from build123d import *

# Parameters (mm, degrees)
SKETCH1_W                   = 54
SKETCH1_H                   = 65
BOSS_EXTRUDE1_DEPTH         = 65
SKETCH2_W                   = 21
SKETCH2_H                   = 41.5
CUT_EXTRUDE1_DEPTH          = 107.611444039
FILLET1_R                   = 6
SKETCH3_W                   = 21
SKETCH3_H                   = 56
CUT_EXTRUDE2_DEPTH          = 32
CUT_EXTRUDE_THIN3_DEPTH     = 9
CUT_EXTRUDE3_DEPTH          = 9
M3_TAPPED_HOLE1_D           = 2.5
M3_TAPPED_HOLE1_CSINK_D     = 3.05
M3_TAPPED_HOLE1_CSINK_ANGLE = 90
HOLE1_D                     = 6.5
HOLE1_CBORE_D               = 11
HOLE1_CBORE_DEPTH           = 7
EXTRUDE_THIN1_START         = 1.5
EXTRUDE_THIN1_DEPTH         = 1.5
M3_TAPPED_HOLE2_D           = 2.5
M3_TAPPED_HOLE2_CSINK_D     = 3.05
M3_TAPPED_HOLE2_CSINK_ANGLE = 90


with BuildPart() as part:
    # Sketch1 → Boss-Extrude1 (new body)
    with BuildSketch(Plane.XY):
        with Locations((27, 32.5)):
            Rectangle(SKETCH1_W, SKETCH1_H)
    extrude(amount=BOSS_EXTRUDE1_DEPTH)

    # Sketch2 → Cut-Extrude1 (cut, through all)
    with BuildSketch(Plane.XY.offset(65)):
        with Locations((27, 32.5)):
            Rectangle(SKETCH2_W, SKETCH2_H)
    extrude(amount=-CUT_EXTRUDE1_DEPTH, mode=Mode.SUBTRACT)

    # Fillet1
    fillet1_edges = [part.edges().sort_by_distance(p)[0] for p in [
        (0, 65, 32.5),
        (0, 0, 32.5),
        (54, 0, 32.5),
        (54, 65, 32.5),
    ]]
    fillet(fillet1_edges, radius=FILLET1_R)

    # Sketch3 → Cut-Extrude2 (cut)
    with BuildSketch(Plane.XY.offset(65)):
        with Locations((27, 32.5)):
            Rectangle(SKETCH3_W, SKETCH3_H)
    extrude(amount=-CUT_EXTRUDE2_DEPTH, mode=Mode.SUBTRACT)

    # Sketch4 → Cut-Extrude-Thin3 (cut)
    with BuildSketch(Plane.XY.offset(65)):
        with BuildLine():
            Line((6.119863014, 48.642808121), (20.863013699, 55.83321895))
            ThreePointArc((20.863013699, 55.83321895), (27, 57.25), (33.136986301, 55.83321895))
            Line((33.136986301, 55.83321895), (47.880136986, 48.642808121))
            ThreePointArc((47.880136986, 48.642808121), (51.25, 43.25), (47.880136986, 37.857191879))
            Line((47.880136986, 37.857191879), (33.136986301, 30.66678105))
            ThreePointArc((33.136986301, 30.66678105), (27, 29.25), (20.863013699, 30.66678105))
            Line((20.863013699, 30.66678105), (6.119863014, 37.857191879))
            ThreePointArc((6.119863014, 37.857191879), (2.75, 43.25), (6.119863014, 48.642808121))
        make_face()
        with BuildLine():
            Line((6.339041096, 48.193407445), (21.082191781, 55.383818273))
            ThreePointArc((21.082191781, 55.383818273), (27, 56.75), (32.917808219, 55.383818273))
            Line((32.917808219, 55.383818273), (47.660958904, 48.193407445))
            ThreePointArc((47.660958904, 48.193407445), (50.75, 43.25), (47.660958904, 38.306592555))
            Line((47.660958904, 38.306592555), (32.917808219, 31.116181727))
            ThreePointArc((32.917808219, 31.116181727), (27, 29.75), (21.082191781, 31.116181727))
            Line((21.082191781, 31.116181727), (6.339041096, 38.306592555))
            ThreePointArc((6.339041096, 38.306592555), (3.25, 43.25), (6.339041096, 48.193407445))
        make_face(mode=Mode.SUBTRACT)
    extrude(amount=-CUT_EXTRUDE_THIN3_DEPTH, mode=Mode.SUBTRACT)

    # Sketch4<3> → Cut-Extrude3 (cut)
    with BuildSketch(Plane.XY.offset(65)):
        with BuildLine():
            Line((32.917808219, 55.383818273), (47.660958904, 48.193407445))
            ThreePointArc((47.660958904, 48.193407445), (50.75, 43.25), (47.660958904, 38.306592555))
            Line((47.660958904, 38.306592555), (32.917808219, 31.116181727))
            ThreePointArc((32.917808219, 31.116181727), (27, 29.75), (21.082191781, 31.116181727))
            Line((21.082191781, 31.116181727), (6.339041096, 38.306592555))
            ThreePointArc((6.339041096, 38.306592555), (3.25, 43.25), (6.339041096, 48.193407445))
            Line((6.339041096, 48.193407445), (21.082191781, 55.383818273))
            ThreePointArc((21.082191781, 55.383818273), (27, 56.75), (32.917808219, 55.383818273))
        make_face()
    extrude(amount=-CUT_EXTRUDE3_DEPTH, mode=Mode.SUBTRACT)

    # M3 Tapped Hole1 (through all)
    with Locations(Plane(origin=(22, 56.85, 33), x_dir=(1, 0, 0), z_dir=(0, 0, 1))):
        with Locations((0, 0), (10, 0), (10, -48.7), (0, -48.7)):
            CounterSinkHole(M3_TAPPED_HOLE1_D / 2, M3_TAPPED_HOLE1_CSINK_D / 2, counter_sink_angle=M3_TAPPED_HOLE1_CSINK_ANGLE)

    # Hole1 (through all)
    with Locations(Plane(origin=(8.25, 56.75, 65), x_dir=(1, 0, 0), z_dir=(0, 0, 1))):
        with Locations((0, 0), (37.5, 0), (37.5, -48.5), (0, -48.5)):
            CounterBoreHole(HOLE1_D / 2, HOLE1_CBORE_D / 2, HOLE1_CBORE_DEPTH)

    # Sketch10 → Extrude-Thin1 (add)
    with BuildSketch(Plane.XY.offset(65).offset(EXTRUDE_THIN1_START)):
        with BuildLine():
            Line((48, 65), (6, 65))
            ThreePointArc((6, 65), (1.757359313, 63.242640687), (0, 59))
            Line((0, 59), (0, 6))
            ThreePointArc((0, 6), (1.757359313, 1.757359313), (6, 0))
            Line((6, 0), (48, 0))
            ThreePointArc((48, 0), (52.242640687, 1.757359313), (54, 6))
            Line((54, 6), (54, 59))
            ThreePointArc((54, 59), (52.242640687, 63.242640687), (48, 65))
        make_face()
        with BuildLine():
            Line((48, 63.5), (6, 63.5))
            ThreePointArc((6, 63.5), (2.818019485, 62.181980515), (1.5, 59))
            Line((1.5, 59), (1.5, 6))
            ThreePointArc((1.5, 6), (2.818019485, 2.818019485), (6, 1.5))
            Line((6, 1.5), (48, 1.5))
            ThreePointArc((48, 1.5), (51.181980515, 2.818019485), (52.5, 6))
            Line((52.5, 6), (52.5, 59))
            ThreePointArc((52.5, 59), (51.181980515, 62.181980515), (48, 63.5))
        make_face(mode=Mode.SUBTRACT)
    extrude(amount=-EXTRUDE_THIN1_DEPTH)

    # M3 Tapped Hole2 (through all)
    with Locations(Plane(origin=(8.25, 24.550881691, 65), x_dir=(1, 0, 0), z_dir=(0, 0, 1))):
        with Locations((0, 0), (37.5, 0)):
            CounterSinkHole(M3_TAPPED_HOLE2_D / 2, M3_TAPPED_HOLE2_CSINK_D / 2, counter_sink_angle=M3_TAPPED_HOLE2_CSINK_ANGLE)


solid = part.part
Geometry: final body of the model. Coordinates: model frame, mm. A direction names the side the tool comes from. Coordinates: 2 decimals unless noted, no trailing zeros. Order: outer loops, then holes, each group sorted by start corner. A loop starts at its lowest first (then second) coordinate and runs counter-clockwise, first axis right, second up. Notation, with made-up numbers: M 75.25,-27 L 111.25,-27 A34 ccw 111.25,3 Z; hole C -26.5,12.5 d8. An arc over 180 degrees is marked long. One line per question, with ' | ' between items. Start each with the question number.
Item 1: Cut plane B-B, the plane y = 30. Return the cut outline in (x, z), then the cut area to 3 significant figures.
Item 2: Draft query along Y for faces 1 (the cylindrical face through (42.65, 9.23, 28.59)), 2 (the flat face through (27, 0, 34)), 3 (the flat face through (0, 33, 34)). Return one class per face: released by +Y, released by -Y, zero draft, split by the parting line, or undercut.
Item 3: Ray query, probe 1 along X at (y, z) = (8.15, 21); probe 2 along Y at (x, z) = (22, 13); probe 3 along Y at (x, z) = (8.25, 28). Return the intervals inside material, ascending. Write a range as [from, to].
Item 4: Cut plane A-A, the plane x = 32. Return the cut outline in (y, z) (3 decimals).
Item 5: Cut plane C-C, the plane x = 26.5. Return the cut outline in (y, z).
Item 6: Pin query (flat end, axial travel): pin 1 Ø4 at (x, y) = (22, 56.85) entering from +Z; pin 2 Ø10.5 at (x, y) = (45.75, 8.25) entering from +Z; pin 3 Ø15 at (x, y) = (44, 47.5) entering from +Z. Return the tip coordinate at first contact, or that it passes through.
Item 7: Set-up query: faces 4 (the flat face through (27, 53.25, 17)), 5 (the flat face through (27, 60.5, 49)). Return all of +Z, -Z, +X, -X, +Y, -Y with unobstructed straight access to the full face (end or side cutting, diameter ignored); none if empty.
Item 8: Cut plane D-D, the plane z = 30. Count the separate pieces of the cut face and the enclosed holes in it, then the cut area to 3 significant figures.
A:
1) outline: M 0,0 L 16.5,0 L 16.5,65 L 1.5,65 L 1.5,66.5 L 0,66.5 Z; M 37.5,0 L 54,0 L 54,66.5 L 52.5,66.5 L 52.5,65 L 37.5,65 Z | area: 2,150 mm2
2) face 1: undercut | face 2: released by -Y | face 3: zero draft
3) probe 1: x = [0, 5], [11.5, 20.75], [23.25, 30.75], [33.25, 42.5], [49, 54] | probe 2: y = [0, 6.9], [9.4, 11.75], [53.25, 55.6], [58.1, 65] | probe 3: y = [0, 5], [11.5, 23.3], [25.8, 53.5], [60, 65]
4) outline: M 0,0 L 6.9,0 L 6.9,32.725 L 6.625,33 L 4.5,33 L 4.5,65 L 1.5,65 L 1.5,66.5 L 0,66.5 Z; M 9.4,0 L 11.75,0 L 11.75,33 L 9.675,33 L 9.4,32.725 Z; M 53.25,0 L 55.6,0 L 55.6,32.725 L 55.325,33 L 53.25,33 Z; M 58.1,0 L 65,0 L 65,66.5 L 63.5,66.5 L 63.5,65 L 60.5,65 L 60.5,33 L 58.375,33 L 58.1,32.725 Z
5) outline: M 0,0 L 11.75,0 L 11.75,33 L 4.5,33 L 4.5,65 L 1.5,65 L 1.5,66.5 L 0,66.5 Z; M 53.25,0 L 65,0 L 65,66.5 L 63.5,66.5 L 63.5,65 L 60.5,65 L 60.5,33 L 53.25,33 Z
6) pin 1: stops at z = 33 | pin 2: stops at z = 58 | pin 3: stops at z = 65
7) face 4: +Z, -Z | face 5: +Z
8) separate pieces: 1 | enclosed holes: 11 | area: 2,450 mm2
